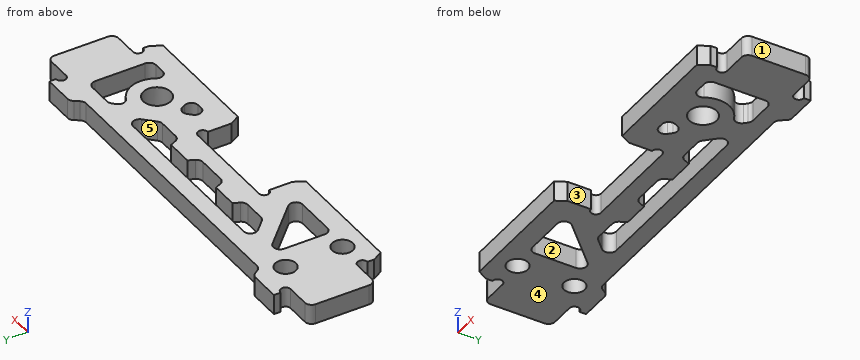
```python
from build123d import *
from OCP.BRepFilletAPI import BRepFilletAPI_MakeChamfer

# Parameters (mm, degrees)
SKETCH_1_R          = 2.05
EXTRUDE_1_DEPTH     = 1.5
SKETCH_2_W          = 4.5
SKETCH_2_H          = 10
EXTRUDE_2_DEPTH     = 3
SKETCH_3_R          = 0.75
CUT_EXTRUDE_1_DEPTH = 51.589030432
FILLET_1_R          = 1
EXTRUDE_3_DEPTH     = 3
CUT_EXTRUDE_2_DEPTH = 51.589030432
FILLET_2_R          = 1
SKETCH_6_R          = 1.55
CUT_EXTRUDE_3_DEPTH = 51.589030432
CUT_EXTRUDE_4_DEPTH = 51.589030432
FILLET_3_R          = 1
CUT_EXTRUDE_5_DEPTH = 51.589030432
FILLET_4_R          = 1
SKETCH_9_W          = 4
SKETCH_9_H          = 1.5
EXTRUDE_4_DEPTH     = 3
CHAMFER_1_SIZE      = 0.699461487
CHAMFER_1_SIZE_2    = 1.5
FILLET_5_R          = 1


with BuildPart() as part:
    # 草图1 → 凸台-拉伸1 (new, symmetric)
    with BuildSketch(Plane.XY):
        Polygon((10, 10), (10, -5), (-10, -5), (-10, 0), (-25, 0), (-25, -5), (-45, -5), (-45, 10), align=None)
        Circle(SKETCH_1_R, mode=Mode.SUBTRACT)
    extrude(amount=EXTRUDE_1_DEPTH, both=True)

    # 草图2 → 凸台-拉伸2 (add)
    with BuildSketch(Plane.XY.offset(1.5)):
        with Locations((12.25, 2.5)):
            Rectangle(SKETCH_2_W, SKETCH_2_H)
        with Locations((-47.25, 2.5)):
            Rectangle(SKETCH_2_W, SKETCH_2_H)
    extrude(amount=-EXTRUDE_2_DEPTH)

    # 草图3 → 切除-拉伸1 (cut, through all)
    with BuildSketch(Plane.XY.offset(1.5)):
        with Locations((-45, 8.25)):
            Circle(SKETCH_3_R)
        with Locations((-45, -3.25)):
            Circle(SKETCH_3_R)
        with Locations((10, 8.25)):
            Circle(SKETCH_3_R)
        with Locations((10, -3.25)):
            Circle(SKETCH_3_R)
        with Locations((-25, -0.75)):
            Circle(SKETCH_3_R)
        with Locations((-10, -0.75)):
            Circle(SKETCH_3_R)
    extrude(amount=-CUT_EXTRUDE_1_DEPTH, mode=Mode.SUBTRACT)

    # 圆角1
    fillet_1_edges = [part.edges().sort_by_distance(p)[0] for p in [
        (14.5, -2.5, 0),
        (14.5, 7.5, 0),
        (-49.5, 7.5, 0),
        (-49.5, -2.5, 0),
    ]]
    fillet(fillet_1_edges, radius=FILLET_1_R)

    # 草图4 → 凸台-拉伸3 (add)
    with BuildSketch(Plane.XY.offset(1.5)):
        Polygon((-10, -5), (-9.133974596, -6.5), (9.133974596, -6.5), (10, -5), align=None)
    extrude_3 = extrude(amount=-EXTRUDE_3_DEPTH)

    # 镜向1: 凸台-拉伸3 across plane
    add(extrude_3.mirror(Plane(origin=(-17.5, 0, 0), x_dir=(0, 0, 1), z_dir=(1, 0, 0))))

    # 草图5 → 切除-拉伸2 (cut, through all)
    with BuildSketch(Plane.XY.offset(1.5)):
        Polygon((-40, 10), (-38.949688693, 8.5), (3.949688693, 8.5), (5, 10), align=None)
    extrude(amount=-CUT_EXTRUDE_2_DEPTH, mode=Mode.SUBTRACT)

    # 圆角2
    fillet_2_edges = [part.edges().sort_by_distance(p)[0] for p in [
        (-40, 10, 0),
        (5, 10, 0),
        (3.949688693, 8.5, 0),
        (-38.949688693, 8.5, 0),
    ]]
    fillet(fillet_2_edges, radius=FILLET_2_R)

    # 草图6 → 切除-拉伸3 (cut, through all)
    with BuildSketch(Plane.XY.offset(1.5)):
        with Locations((-40.5, 5.5)):
            Circle(SKETCH_6_R)
        with Locations((-40.5, -3)):
            Circle(SKETCH_6_R)
    extrude(amount=-CUT_EXTRUDE_3_DEPTH, mode=Mode.SUBTRACT)

    # 草图7 → 切除-拉伸4 (cut, through all)
    with BuildSketch(Plane.XY.offset(1.5)):
        Polygon((-37, 6), (-37, -3.5), (-27.5, -3.5), align=None)
        Polygon((-33.464466094, 6), (-1.535533906, 6), (-5.035533906, 2.5), (-29.964466094, 2.5), align=None)
    extrude(amount=-CUT_EXTRUDE_4_DEPTH, mode=Mode.SUBTRACT)

    # 圆角3
    fillet_3_edges = [part.edges().sort_by_distance(p)[0] for p in [
        (-29.964466094, 2.5, 0),
        (-33.464466094, 6, 0),
        (-1.535533906, 6, 0),
        (-5.035533906, 2.5, 0),
        (-37, 6, 0),
        (-27.5, -3.5, 0),
        (-37, -3.5, 0),
    ]]
    fillet(fillet_3_edges, radius=FILLET_3_R)

    # 草图8 → 切除-拉伸5 (cut, through all)
    with BuildSketch(Plane.XY.offset(1.5)):
        with BuildLine():
            Line((7, 6), (7, -3.5))
            Line((7, -3.5), (1.936491673, -3.5))
            ThreePointArc((1.936491673, -3.5), (3.872983346, 1), (0, 4))
            Line((0, 4), (2, 6))
            Line((2, 6), (7, 6))
        make_face()
        with BuildLine():
            Line((-1.936491673, -3.5), (-7.5, -3.5))
            Line((-7.5, -3.5), (-4, 0))
            ThreePointArc((-4, 0), (-3.445719569, -2.031506006), (-1.936491673, -3.5))
        make_face()
    extrude(amount=-CUT_EXTRUDE_5_DEPTH, mode=Mode.SUBTRACT)

    # 圆角4
    fillet_4_edges = [part.edges().sort_by_distance(p)[0] for p in [
        (2, 6, 0),
        (7, 6, 0),
        (7, -3.5, 0),
        (1.936491673, -3.5, 0),
        (0, 4, 0),
        (-4, 0, 0),
        (-1.936491673, -3.5, 0),
        (-7.5, -3.5, 0),
    ]]
    fillet(fillet_4_edges, radius=FILLET_4_R)

    # 草图9 → 凸台-拉伸4 (add)
    with BuildSketch(Plane.XY.offset(1.5)):
        with Locations((-23, 3.25)):
            Rectangle(SKETCH_9_W, SKETCH_9_H)
        with Locations((-12, 3.25)):
            Rectangle(SKETCH_9_W, SKETCH_9_H)
    extrude(amount=-EXTRUDE_4_DEPTH)

    # 倒角1
    chamfer_1_edges_1 = [part.edges().sort_by_distance(p)[0] for p in [
        (-14, 2.5, 0),
    ]]
    chamfer_1_side_1 = [part.faces().sort_by_distance(p)[0] for p in [
        (-14.01398923, 2.5, 0),
    ]]
    chamfer_1_edges_2 = [part.edges().sort_by_distance(p)[0] for p in [
        (-10, 2.5, 0),
    ]]
    chamfer_1_side_2 = [part.faces().sort_by_distance(p)[0] for p in [
        (-9.98601077, 2.5, 0),
    ]]
    chamfer_1_edges_3 = [part.edges().sort_by_distance(p)[0] for p in [
        (-21, 2.5, 0),
    ]]
    chamfer_1_side_3 = [part.faces().sort_by_distance(p)[0] for p in [
        (-20.98601077, 2.5, 0),
    ]]
    chamfer_1_edges_4 = [part.edges().sort_by_distance(p)[0] for p in [
        (-25, 2.5, 0),
    ]]
    chamfer_1_side_4 = [part.faces().sort_by_distance(p)[0] for p in [
        (-25.01398923, 2.5, 0),
    ]]
    chamfer_1 = BRepFilletAPI_MakeChamfer(part.part.solid().wrapped)
    for e in chamfer_1_edges_1:
        chamfer_1.Add(CHAMFER_1_SIZE - 0.0001, CHAMFER_1_SIZE_2 - 0.0001, e.wrapped, chamfer_1_side_1[0].wrapped)
    for e in chamfer_1_edges_2:
        chamfer_1.Add(CHAMFER_1_SIZE - 0.0001, CHAMFER_1_SIZE_2 - 0.0001, e.wrapped, chamfer_1_side_2[0].wrapped)
    for e in chamfer_1_edges_3:
        chamfer_1.Add(CHAMFER_1_SIZE - 0.0001, CHAMFER_1_SIZE_2 - 0.0001, e.wrapped, chamfer_1_side_3[0].wrapped)
    for e in chamfer_1_edges_4:
        chamfer_1.Add(CHAMFER_1_SIZE - 0.0001, CHAMFER_1_SIZE_2 - 0.0001, e.wrapped, chamfer_1_side_4[0].wrapped)
    add(Compound.cast(chamfer_1.Shape()), mode=Mode.REPLACE)  # a hair under: the kernel refuses the full size

    # 圆角5
    fillet_5_edges = [part.edges().sort_by_distance(p)[0] for p in [
        (-20.300638513, 2.5, 0),
        (-14.699361487, 2.5, 0),
        (-9.300638513, 2.5, 0),
        (-25.699361487, 2.5, 0),
    ]]
    fillet(fillet_5_edges, radius=FILLET_5_R)


solid = part.part
```
CAD build for the part. Positions are in the model's coordinates, mm. Face numbers are marked on the shaded views. A direction names the side the tool comes from. Round coordinates to 2 decimals unless told otherwise and drop trailing zeros. Order: outer loops, then holes, each group sorted by start corner. A loop starts at its lowest first (then second) coordinate and runs counter-clockwise, first axis right, second up.
Item 1: Tool access for the marked faces 1, 2 and 3: list every direction of +Z, -Z, +X, -X, +Y, -Y with a clear straight run to the whole face (end or side of a thin tool).
Item 2: Mould opens along Y. For the marked faces 4 and 5 say: pulls with the +Y half, pulls with the -Y half, needs draft (parallel to the pull), parting line crosses it, or undercut.
Item 3: Saw through at C-C on z = 0. State how many separate pieces and enclosed holes the cut face has, then the cut area to 3 significant figures.
Item 4: Pin check, flat tips, straight feed: pin 1 (0.9 mm diameter, centred on x = -24, z = 0, fed in from -Y); pin 2 (0.5 mm diameter, centred on x = 5, z = 0, fed in from +Y); pin 3 (1.5 mm diameter, centred on y = 7.5, z = -1, fed in from -X). Stop position of each tip, or through.
Item 5: Saw through at A-A on x = -41.5. Write the cut outline in (y, z).
Item 6: Saw through at B-B on x = -1. Write the cut outline in (y, z).
Item 7: Probe line 1 along Y through (x, z) = (-40.5, 0.7); line 2 along Y through (x, z) = (0, -0.5); line 3 along X through (y, z) = (-0.75, 0.2). List the from-to ranges inside material, lowest first.
Reported:
1. face 1: +Z, -Z, +X, +Y, -Y
1. face 2: +Z, -Z
1. face 3: +Z, -Z, -Y
2. face 4: needs draft
2. face 5: undercut
3. separate pieces: 1
3. enclosed holes: 7
3. area: 629 mm2
4. pin 1: stops at y = 0
4. pin 2: stops at y = 9.96
4. pin 3: stops at x = -49.47
5. outline: (-6.5, -1.5) - (-4.18, -1.5) - (-4.18, 1.5) - (-6.5, 1.5) - close; (-1.82, -1.5) - (4.32, -1.5) - (4.32, 1.5) - (-1.82, 1.5) - close; (6.68, -1.5) - (10, -1.5) - (10, 1.5) - (6.68, 1.5) - close
6. outline: (-6.5, -1.5) - (-1.79, -1.5) - (-1.79, 1.5) - (-6.5, 1.5) - close; (1.79, -1.5) - (8.5, -1.5) - (8.5, 1.5) - (1.79, 1.5) - close
7. line 1: y = -6.5 to -4.55, -1.45 to 3.95, 7.05 to 10
7. line 2: y = -6.5 to -2.05, 2.05 to 8.5
7. line 3: x = -49.5 to -37, -30.25 to -25.75, -9.25 to -1.91, 1.91 to 3.93, 7 to 14.5
